Verification items for the finished model (mm, model axes). Coordinates: 2 decimals unless noted, no trailing zeros. Loops run counter-clockwise (first coordinate to the right, second up) from the corner with the lowest first, then second, coordinate; pieces in that order, holes last. Notation, with made-up numbers: (51.5, 43.5) - (99.5, 43.5) arc R7 ccw to (99.5, 50.5) - close; hole circle Ø6 at (15, 17.25). An arc over 180 degrees is marked (long way). Answer as CSV lines item,"result". Start each with the question number.
1. Cross-section at B-B (x = 32). Enter the section's corners in (y, z), plus the area to 3 significant figures.
2. Material ranges on line 1 (Y direction, x = 32, z = 2.1); line 2 (X direction, y = 10, z = 0.8); line 3 (Y direction, x = 10, z = 2.1), recorded low to high. Write a range as [from, to].
3. Cross-section at D-D (z = 1.55). Enter the section's corners in (x, y).
4. Gauge pin test, flat ends, axial feed: P1, Ø1.8, axis at x = 32, y = 32, coming from the -Z side; P2, Ø1.5, axis at x = 22.5, z = 1, coming from the +Y side; P3, Ø1.5, axis at y = 29.5, z = 2, coming from the -X side. Record the tip position at first contact, or that the pin passes through.
5. Cross-section at C-C (y = 10). Enter the section's corners in (x, z), plus the area to 3 significant figures.
6. Cross-section at A-A (x = 10). Enter the section's corners in (y, z), plus the area to 3 significant figures.
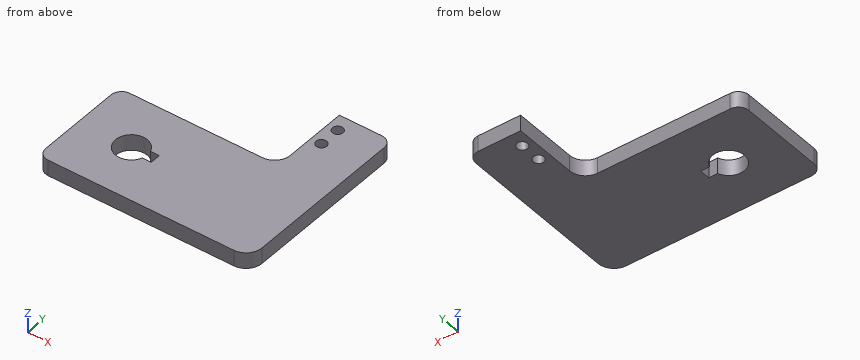
Autodesk Inventor part; units mm, degrees
ref_plane "YZ Plane" through (0, 0, 0) normal (1, 0, 0) x (0, 1, 0)
ref_plane "XZ Plane" through (0, 0, 0) normal (0, 1, 0) x (-1, 0, 0)
ref_plane "XY Plane" through (0, 0, 0) normal (0, 0, 1) x (1, 0, 0)
sketch "スケッチ1" plane through (0, 0, 0) normal (0, 0, 1) x (1, 0, 0)
  line L0 (0, 0) -> (0, 20)
  line L1 (0, 0) -> (40, 0)
  line L2 (40, 0) -> (40, 35)
  line L3 (40, 35) -> (30, 35)
  line L4 (30, 35) -> (30, 20)
  line L5 (30, 20) -> (0, 20)
  circle A0 centre (10, 10) radius 3
  line L6 (10, 10) -> (10, 9)
  line L7 (10, 10) -> (10, 11)
  line L8 (10, 9) -> (14.5, 9)
  line L9 (14.5, 9) -> (14.5, 11)
  line L10 (14.5, 11) -> (10, 11)
  point P0 (12.8284, 9)
  point P1 (12.8284, 11)
  dimension "d0" = 20
  dimension "d1" = 40
  dimension "d2" = 35
  dimension "d3" = 10
  dimension "d4" = 6
  dimension "d6" = 1
  dimension "d7" = 1
  dimension "d8" = 4.5
extrude "押し出し1" add sketch "スケッチ1" along normal blind 3
fillet "フィレット1" radius 3 2 edges at (30, 20, 1.5) (40, 0, 1.5)
fillet "フィレット2" radius 2 2 edges at (0, 20, 1.5) (0, 0, 1.5)
fillet "フィレット3" radius 2 1 edges at (40, 35, 1.5)
sketch "スケッチ3" plane through (0, 0, 3) normal (0, 0, 1) x (1, 0, 0)
  circle A0 centre (32, 28) radius 1
  circle A1 centre (32, 32) radius 1
  point P0 (0, 0)
  dimension "d23" = 2
  dimension "d24" = 2
extrude "押し出し3" cut sketch "スケッチ3" against normal blind 10
thread "ねじ3"
thread "ねじ4"
properties part number "cutter_holder" material "アルミニウム 7075"
Values follow:
1,outline,"(0, 0) - (27, 0) - (27, 3) - (0, 3) - close; (29, 0) - (31, 0) - (31, 3) - (29, 3) - close; (33, 0) - (35, 0) - (35, 3) - (33, 3) - close"
1,area,"93.0 mm²"
2,line 1,"y = [0, 27], [29, 31], [33, 35]"
2,line 2,"x = [0, 7], [14.5, 40]"
2,line 3,"y = [0, 7], [13, 20]"
3,outline,"(0, 2) arc R2 ccw to (2, 0) - (37, 0) arc R3 ccw to (40, 3) - (40, 33) arc R2 ccw to (38, 35) - (30, 35) - (30, 23) arc R3 cw to (27, 20) - (2, 20) arc R2 ccw to (0, 18) - close; hole (12.83, 9) - (14.5, 9) - (14.5, 11) - (12.83, 11) arc R3 ccw (long way) to start; hole circle Ø2 at (32, 28); hole circle Ø2 at (32, 32)"
4,P1,"passes through"
4,P2,"stops at y = 20"
4,P3,"stops at x = 30"
5,outline,"(0, 0) - (7, 0) - (7, 3) - (0, 3) - close; (14.5, 0) - (40, 0) - (40, 3) - (14.5, 3) - close"
5,area,"97.5 mm²"
6,outline,"(0, 0) - (7, 0) - (7, 3) - (0, 3) - close; (13, 0) - (20, 0) - (20, 3) - (13, 3) - close"
6,area,"42.0 mm²"
